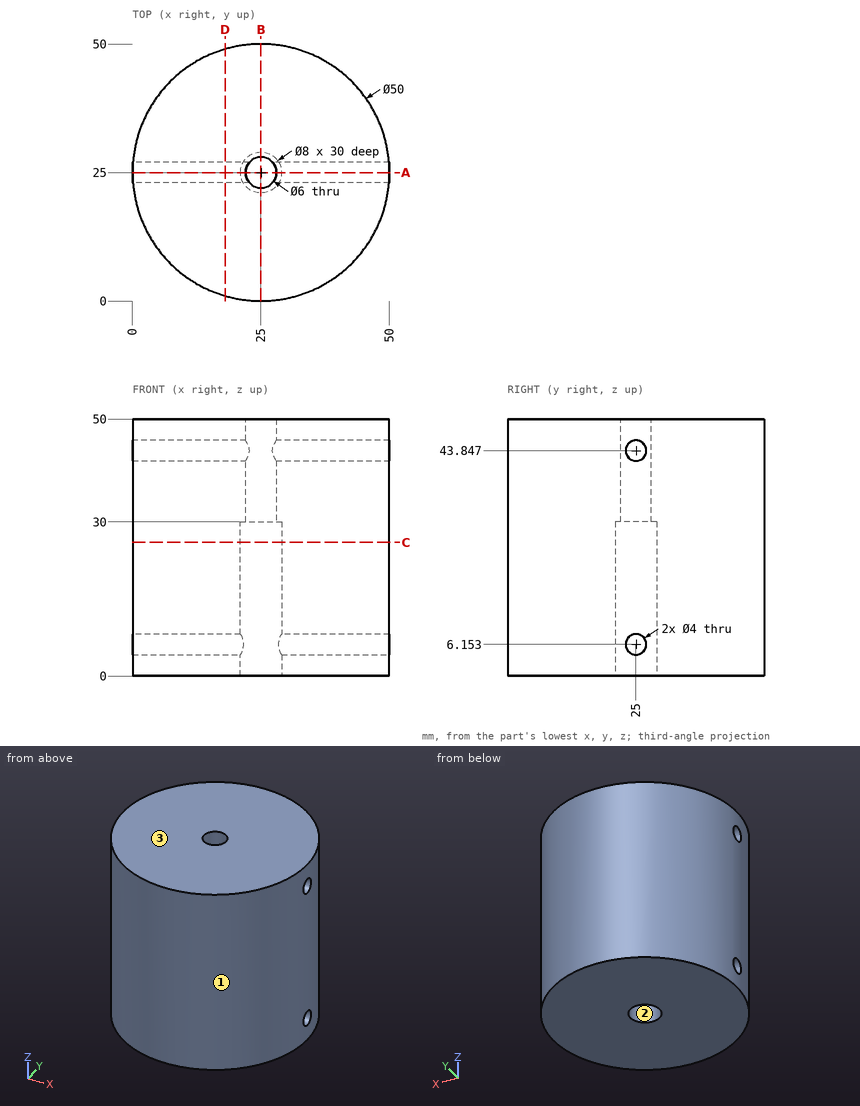
Input: dimensioned drawing with shaded views. Units: mm. Origin: part minimum x, y, z. Round coordinates to 2 decimals unless told otherwise and drop trailing zeros. Write each loop counter-clockwise with the first axis right and the second up, starting at its lowest first coordinate (ties: lowest second). Pieces come first, ordered by that corner, then holes. Notation, with made-up numbers: (34, 60) -> (54, 60) arc R29 cw to (54, 96) -> close; hole circle Ø8 at (22, 38.25). An arc over 180 degrees is marked (long way). Use CSV: the item, a comma, the result in double quotes. Start each with the question number.
Q1. Section A-A (y = 25). Return loops of the section in (x, z).
Q2. Line query: L1, parallel to Y at x = 25, z = 37.5; L2, parallel to Y at x = 25, z = 9.5; L3, parallel to Z at x = 34, y = 26.5 (1 decimal). Output: solid intervals per line, ascending.
Q3. Section B-B (x = 25). Return loops of the section in (y, z), plus the area to 3 significant figures.
Q4. Section D-D (x = 18). Return loops of the section in (y, z), plus the area to 4 significant figures.
Q5. First-contact query: pin 1 Ø1.5 at (y, z) = (31.5, 23) entering from -X; pin 2 Ø4 at (y, z) = (17, 28) entering from +X; pin 3 Ø2 at (x, y) = (44.5, 42.5) entering from -Z; pin 4 Ø4 at (y, z) = (36, 7.5) entering from +X. Flat tips, straight axial feed; report the tip coordinate or a pass-through.
Q6. Pull-direction query (Y, two-part tool) for the marked faces 1, 2 and 3; classes: pulls with the +Y half, pulls with the -Y half, needs draft (parallel to the pull), parting line crosses it, or undercut.
Q7. Section C-C (z = 26). Return loops of the section in (x, y).
Result sheet:
1,outline,"(0, 0) -> (21, 0) -> (21, 4.15) -> (0, 4.15) -> close; (0, 8.15) -> (21, 8.15) -> (21, 30) -> (22, 30) -> (22, 41.85) -> (0, 41.85) -> close; (0, 45.85) -> (22, 45.85) -> (22, 50) -> (0, 50) -> close; (28, 30) -> (29, 30) -> (29, 8.15) -> (50, 8.15) -> (50, 41.85) -> (28, 41.85) -> close; (28, 45.85) -> (50, 45.85) -> (50, 50) -> (28, 50) -> close; (29, 0) -> (50, 0) -> (50, 4.15) -> (29, 4.15) -> close"
2,L1,"0 to 22, 28 to 50"
2,L2,"0 to 21, 29 to 50"
2,L3,"0 to 4.8, 7.5 to 42.5, 45.2 to 50"
3,outline,"(0, 0) -> (21, 0) -> (21, 30) -> (22, 30) -> (22, 50) -> (0, 50) -> close; (28, 30) -> (29, 30) -> (29, 0) -> (50, 0) -> (50, 50) -> (28, 50) -> close"
3,area,"2,140 mm²"
4,outline,"(1, 0) -> (49, 0) -> (49, 50) -> (1, 50) -> close; hole circle Ø4 at (25, 6.15); hole circle Ø4 at (25, 43.85)"
4,area,"2,375 mm²"
5,pin 1,"x = 0.67"
5,pin 2,"x = 49.27"
5,pin 3,"through"
5,pin 4,"x = 48.32"
6,face 1,"parting line crosses it"
6,face 2,"undercut"
6,face 3,"needs draft"
7,outline,"circle Ø50 at (25, 25); hole circle Ø8 at (25, 25)"
